```python
from build123d import *

# Parameters (mm, degrees)
SKETCH1_W           = 90.7
SKETCH1_H           = 7.2
SKETCH1_R           = 1.5
BOSS_EXTRUDE1_DEPTH = 3.8
FILLET1_R           = 1


with BuildPart() as part:
    # Sketch1 → Boss-Extrude1 (new body)
    with BuildSketch(Plane(origin=(0, 0, 0), x_dir=(1, 0, 0), z_dir=(0, 1, 0))):
        Rectangle(SKETCH1_W, SKETCH1_H)
        with Locations(Location((-41.35, -0.1, 0), (0, 0, 90))):
            Circle(SKETCH1_R, mode=Mode.SUBTRACT)
        with Locations(Location((0.05, -0.1, 0), (0, 0, 90))):
            Circle(SKETCH1_R, mode=Mode.SUBTRACT)
        with Locations(Location((41.35, -0.1, 0), (0, 0, 90))):
            Circle(SKETCH1_R, mode=Mode.SUBTRACT)
    extrude(amount=BOSS_EXTRUDE1_DEPTH)

    # Fillet1
    fillet1_edges = [part.edges().sort_by_distance(p)[0] for p in [
        (45.35, 3.8, 0),
        (0, 3.8, -3.6),
        (-45.35, 3.8, 0),
        (0, 0, -3.6),
        (45.35, 0, 0),
        (0, 0, 3.6),
        (-45.35, 0, 0),
        (-45.35, 1.9, -3.6),
        (45.35, 1.9, -3.6),
        (45.35, 1.9, 3.6),
        (-45.35, 1.9, 3.6),
        (0, 3.8, 3.6),
    ]]
    fillet(fillet1_edges, radius=FILLET1_R)


solid = part.part
```
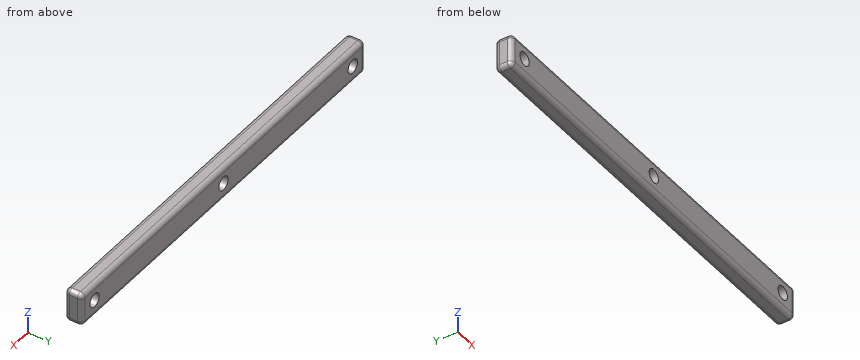
Here's how the part is built. I have some questions about the finished solid (model axes, mm). Give positions to 0.01 mm unless a question says otherwise; leave off trailing zeros. Loops run counter-clockwise (first coordinate to the right, second up) from the corner with the lowest first, then second, coordinate; pieces in that order, holes last. Notation, with made-up numbers: M 60.25,7.5 L 103.25,7.5 A23 ccw 103.25,24.5 Z; hole C 72,-29.5 d6. An arc over 180 degrees is marked long. Return JSON: item names as keys, results as strings.
Item 1: Imagine slicing it at A-A on z = 0.1. List the corners of the cut face in (x, y) for me, then the cut area to 3 significant figures.
A:
{"outline": "M -45.35,1 A1 ccw -44.35,0 L -42.85,0 L -42.85,3.8 L -44.35,3.8 A1 ccw -45.35,2.8 Z; M -39.85,0 L -1.45,0 L -1.45,3.8 L -39.85,3.8 Z; M 1.55,0 L 39.85,0 L 39.85,3.8 L 1.55,3.8 Z; M 42.85,0 L 44.35,0 A1 ccw 45.35,1 L 45.35,2.8 A1 ccw 44.35,3.8 L 42.85,3.8 Z", "area": "310 mm^2"}
Item 2: I'm going to push flat-ended pins straight in: pin 1 Ø1 at (x, y) = (29, 0.5) entering from +Z; pin 2 Ø2.5 at (x, z) = (41.35, 0.1) entering from +Y. Where does each tip first touch, or does it pass through?
A:
{"pin 1": "stops at z = 3.6", "pin 2": "passes through"}
Item 3: Imagine slicing it at C-C on x = 18. List the corners of the cut face in (y, z) for me, then the cut area to 3 significant figures.
A:
{"outline": "M 0,-2.6 A1 ccw 1,-3.6 L 2.8,-3.6 A1 ccw 3.8,-2.6 L 3.8,2.6 A1 ccw 2.8,3.6 L 1,3.6 A1 ccw 0,2.6 Z", "area": "26.5 mm^2"}
Item 4: Imagine slicing it at B-B on x = 0.05. List the corners of the cut face in (y, z) for me.
A:
{"outline": "M 0,-2.6 A1 ccw 1,-3.6 L 2.8,-3.6 A1 ccw 3.8,-2.6 L 3.8,-1.4 L 0,-1.4 Z; M 0,1.6 L 3.8,1.6 L 3.8,2.6 A1 ccw 2.8,3.6 L 1,3.6 A1 ccw 0,2.6 Z"}
Item 5: Please list where these lines run through material, in increasing order: line 1 (X direction, y = 2.45, z = 0.1); line 2 (Z direction, x = 41.35, y = 2.95); line 3 (X direction, y = 3.65, z = 1).
A:
{"line 1": "x = -45.35 to -42.85, -39.85 to -1.45, 1.55 to 39.85, 42.85 to 45.35", "line 2": "z = -3.59 to -1.4, 1.6 to 3.59", "line 3": "x = -44.88 to -42.55, -40.15 to -1.15, 1.25 to 40.15, 42.55 to 44.88"}
